Autodesk Inventor part; units mm, degrees
ref_plane "作業平面1" through (0, 0, 14) normal (0, 0, 1) x (-0.9659, -0.2588, 0)
ref_plane "YZ Plane" through (0, 0, 0) normal (1, 0, 0) x (0, 1, 0)
ref_plane "XZ Plane" through (0, 0, 0) normal (0, 1, 0) x (-1, 0, 0)
ref_plane "作業平面1" through (0, 0, 14) normal (0, 0, 1) x (-0.9659, -0.2588, 0)
sketch "スケッチ14" plane through (0, 0, 0) normal (0, 0, 1) x (1, 0, 0)
  circle A0 centre (0, 0) radius 25
  circle A1 centre (30, 0) radius 4.05
  line L0 (0, 25) -> (40, 25)
  line L1 (40, 25) -> (40, -25)
  line L2 (40, -25) -> (0, -25)
  line L3 (0, -25) -> (0, 25)
  line L4 (0, -25) -> (40, -10.4412)
  line L5 (0, 25) -> (40, 10.4412)
  line L6 (0.5157, 26.4168) -> (40.5157, 11.858)
  line L7 (0.5157, -26.4168) -> (40.5157, -11.858)
  circle A2 centre (0, 0) radius 6.5
  circle A3 centre (0, 0) radius 28
  line L8 (1.5417, 29.2358) -> (41.5417, 14.677)
  line L9 (1.5417, -29.2358) -> (41.5417, -14.677)
  point P0 (8.5505, -23.4923)
  point P1 (40, -12.0456)
  point P2 (40, 12.0456)
  point P3 (8.5505, 23.4923)
  point P4 (40, 15.2382)
  point P5 (9.5766, 26.3114)
  point P6 (9.5766, -26.3114)
  point P7 (40, -15.2382)
  dimension "d111" = 50
  dimension "d112" = 8.1
  dimension "d113" = 30
  dimension "d114" = 40
  dimension "d115" = 50
  dimension "d116" = 25
  dimension "d119" = 25
  dimension "d126" = 20
  dimension "d127" = 20
  dimension "d144" = 13
  dimension "d207" = 3
  dimension "d208" = 3
  dimension "d209" = 3
extrude "押し出し9" add sketch "スケッチ14" along normal blind 5 contours L3 A2 A0 | L0 L6 A0 | A0 L2 A3 L0 | L5 A0 L4 L3 A2 | A0 L5 | L4 A0 | A0 L7 L2 | L6 A3 L5 A0 | L6 L0 A3 | L5 A3 A1 L4 A0 | L7 A3 L2 | A0 L4 A3 L7 | A3 L0 L8 L1 L6 | L6 L1 L5 A3 | A3 L8 L0 | L5 L1 L4 A3 A1 | A3 L4 L1 L7 | L7 L1 L9 L2 A3 | L2 L9 A3
sketch "スケッチ15" plane through (0, 0, 0) normal (0, 0, -1) x (-1, 0, 0)
  circle A0 centre (-30, 0) radius 4.05
  circle A1 centre (-30, 0) radius 6.6
  point P0 (0, 0)
  dimension "d122" = 13.2
extrude "押し出し10" cut sketch "スケッチ15" against normal blind 2
sketch "スケッチ16" plane through (0, 0, 5) normal (0, 0, 1) x (1, 0, 0)
  circle A0 centre (30, 0) radius 4.05
  circle A1 centre (30, 0) radius 17
  arc A2 (8.5505, 23.4923) -> (8.5505, -23.4923) centre (0, 0) ccw
  circle A3 centre (0, 0) radius 25
  line L0 (40, -15.2382) -> (40, 15.2382)
  line L1 (40, 12.0456) -> (-0.2187, 26.6841)
  line L2 (40, -12.0456) -> (-2.6962, -27.5858)
  circle A4 centre (0, 0) radius 17.5
  line L3 (8.5505, 23.4923) -> (5.9854, 16.4446)
  line L4 (-17.5, 0) -> (-25, 0)
  line L5 (-2.7839, 19.6364) -> (32.5, 6.7941)
  line L6 (32.5, 6.7941) -> (32.5, -6.7941)
  line L7 (32.5, -6.7941) -> (-5.2613, -20.5381)
  line L8 (17.9474, 20.0721) -> (15.3823, 13.0244)
  point P0 (0, 25)
  point P1 (0, -25)
  dimension "d125" = 34
  dimension "d128" = 7.5
  dimension "d164" = 7.5
  dimension "d165" = 10
extrude "押し出し11" add sketch "スケッチ16" along normal blind 10 contours L8 L5 L3 A3 | A3 L1 L8 | L3 A4 L4 A2
sketch "スケッチ17" plane through (0, 0, 5) normal (0, 0, 1) x (1, 0, 0)
  circle A0 centre (30, 0) radius 4.05
  line L0 (0, 0) -> (30, 0)
  circle A1 centre (0, 0) radius 12.5
  line L1 (0, 0) -> (12.4415, 7.1831)
  point P0 (10.8253, 6.25)
  point P1 (0, 12.5)
  point P2 (-10.8253, 6.25)
  point P3 (-10.8253, -6.25)
  point P4 (0, -12.5)
  point P5 (10.8253, -6.25)
  dimension "d131" = 25
  dimension "d132" = 30
  dimension "d135" = 360
hole "穴5" at (10.8253, 6.25, 5) at (0, 12.5, 5) at (-10.8253, 6.25, 5) at (-10.8253, -6.25, 5) at (0, -12.5, 5) at (10.8253, -6.25, 5) direction (0, 0, -1) diameter 3.2 end through all
sketch "スケッチ18" plane through (0, 0, 5) normal (0, 0, 1) x (1, 0, 0)
  circle A0 centre (30, 0) radius 4.05
  line L0 (0, 0) -> (30, 0)
  circle A1 centre (0, 0) radius 10.2
  point P0 (10.2, 0)
  point P1 (-5.1, 8.8335)
  point P2 (-5.1, -8.8335)
  dimension "d145" = 20.4
  dimension "d148" = 360
hole "穴6" at (10.2, 0, 5) at (-5.1, 8.8335, 5) at (-5.1, -8.8335, 5) direction (0, 0, -1) diameter 4.2 end through all
sketch "スケッチ19" plane through (0, 0, 5) normal (0, 0, 1) x (1, 0, 0)
  circle A0 centre (0, 12.5) radius 1.6
  circle A1 centre (0, 0) radius 12.5
  circle A2 centre (0, 12.5) radius 3
  circle A3 centre (-10.8253, 6.25) radius 3
  circle A4 centre (-10.8253, -6.25) radius 3
  circle A5 centre (0, -12.5) radius 3
  circle A6 centre (10.8253, -6.25) radius 3
  circle A7 centre (10.8253, 6.25) radius 3
  dimension "d157" = 6
  dimension "d160" = 360
extrude "押し出し12" cut sketch "スケッチ19" against normal blind 3 contours A0 A1 | A0 A1 A2 | A1 A0 | A0 A1 A2 | A3 A1 | A1 A3 | A7 A1 | A1 A7 | A4 A1 | A1 A4 | A6 A1 | A1 A6 | A5 A1 | A1 A5
sketch "スケッチ20" plane through (0, 0, 15) normal (0, 0, 1) x (1, 0, 0)
  line L0 (17.9474, 20.0721) -> (8.5505, 23.4923)
  line L1 (17.9474, 20.0721) -> (15.3823, 13.0244)
  line L2 (15.3823, 13.0244) -> (5.9854, 16.4446)
  line L3 (5.9854, 16.4446) -> (8.5505, 23.4923)
  line L4 (0, 0) -> (0, 30.7788)
  circle A0 centre (0, 0) radius 21.25
  circle A1 centre (0, 0) radius 25
  point P0 (11.9664, 18.2584)
  point P1 (0, 21.25)
  point P2 (-10.625, 18.403)
  point P3 (-18.403, 10.625)
  point P4 (-21.25, 0)
  point P5 (-18.403, -10.625)
  point P6 (-10.625, -18.403)
  point P7 (0, -21.25)
  point P8 (10.625, -18.403)
  point P9 (18.403, -10.625)
  point P10 (21.25, 0)
  point P11 (18.403, 10.625)
  point P12 (10.625, 18.403)
  dimension "d167" = 7.5
  dimension "d168" = 5
  dimension "d169" = 3.75
  dimension "d170" = 3.75
  dimension "d171" = 50
  dimension "d174" = 360
hole "穴7" at (11.9664, 18.2584, 15) at (0, 21.25, 15) at (-10.625, 18.403, 15) at (-18.403, 10.625, 15) direction (0, 0, -1) diameter 2.459 end through all
sketch "スケッチ21" plane through (0, 0, 15) normal (0, 0, 1) x (1, 0, 0)
  circle A0 centre (0, 0) radius 25
  line L0 (40, -15.2382) -> (40, 15.2382)
  line L1 (40, 12.0456) -> (40, -12.0456)
  line L2 (8.5505, -23.4923) -> (40, -12.0456)
  line L3 (40, -12.0456) -> (8.5505, -23.4923)
  line L4 (40, 12.0456) -> (8.5505, 23.4923)
  line L5 (40, 0) -> (-25, 0)
  circle A1 centre (0, 0) radius 16
  circle A2 centre (30, 0) radius 4.05
  circle A3 centre (30, 0) radius 4.05
  line L6 (9.2345, 25.3717) -> (42, 13.4461)
  line L7 (42, 13.4461) -> (42, -13.4461)
  line L8 (42, -13.4461) -> (9.2345, -25.3717)
  circle A4 centre (0, 0) radius 27
  line L9 (40, 15.2382) -> (40, -15.2382)
  point P0 (40, 14.174)
  point P1 (9.2345, 25.3717)
  point P2 (9.2345, -25.3717)
  point P3 (40, -14.174)
  dimension "d183" = 32
  dimension "d184" = 8.1
  dimension "d210" = 2
  dimension "d211" = 2
extrude "押し出し13" add sketch "スケッチ21" along normal blind 5 contours L5 A1 A0 | L5 A2 A4 L2 A0 | A0 L5 A1 | A0 L4 A4 A2 L5 | A0 L2 A4 L4 | A4 L6 L0 L4 | L4 L0 L5 A2 A4 | A4 A2 L5 L0 L2 | L2 L0 L8 A4
sketch "スケッチ22" plane through (0, 0, 20) normal (0, 0, 1) x (1, 0, 0)
  circle A0 centre (0, 21.25) radius 1.2295
  circle A1 centre (0, 0) radius 21.25
  circle A2 centre (-10.625, 18.403) radius 1.2295
  circle A3 centre (-18.403, 10.625) radius 1.2295
  circle A4 centre (11.9664, 18.2584) radius 1.2295
  line L0 (-17.5, 0) -> (-25, 0)
  line L1 (-25, 0) -> (40, 0)
  line L2 (40, -15.2382) -> (40, 15.2382)
  point P0 (40, -12.0456)
  point P1 (40, 12.0456)
  point P2 (0, -21.25)
  point P3 (-10.625, -18.403)
  point P4 (-18.403, -10.625)
  point P5 (11.9664, -18.2584)
  point P6 (-21.25, 0)
  point P7 (-18.403, 10.625)
  point P8 (-21.25, 0)
  point P9 (-18.403, -10.625)
  point P10 (-10.625, -18.403)
  point P11 (0, -21.25)
  point P12 (10.625, -18.403)
  point P13 (18.403, -10.625)
  point P14 (21.25, 0)
  point P15 (18.403, 10.625)
  point P16 (10.625, 18.403)
  point P17 (0, 21.25)
  dimension "d215" = 360
hole "穴8" at (10.625, -18.403, 20) at (0, -21.25, 20) at (-10.625, -18.403, 20) at (-18.403, -10.625, 20) at (-18.403, 10.625, 20) at (-21.25, 0, 20) at (-10.625, 18.403, 20) at (0, 21.25, 20) at (10.625, 18.403, 20) direction (0, 0, -1) diameter 3.2 end through all
sketch "スケッチ23" plane through (0, 0, 0) normal (0, 0, -1) x (-1, 0, 0)
  line L0 (46.3543, -34.5724) -> (-56.544, -34.5724)
  line L1 (-56.544, -34.5724) -> (-56.544, 32.2069)
  line L2 (-56.544, 32.2069) -> (46.3543, 32.2069)
  line L3 (46.3543, 32.2069) -> (46.3543, -34.5724)
  point P0 (0, 0)
extrude "押し出し14" cut sketch "スケッチ23" against normal blind 15
sketch "スケッチ24" plane through (0, 0, 20) normal (0, 0, 1) x (1, 0, 0)
  circle A0 centre (0, 21.25) radius 1.6
  circle A1 centre (0, 21.25) radius 3
  circle A2 centre (-10.625, 18.403) radius 1.6
  circle A3 centre (-10.625, 18.403) radius 3
  circle A4 centre (-18.403, 10.625) radius 1.6
  circle A5 centre (-18.403, 10.625) radius 3
  line L0 (0, 0) -> (-8.2063, 0)
  circle A6 centre (0, -21.25) radius 3
  circle A7 centre (-10.625, -18.403) radius 3
  circle A8 centre (-18.403, -10.625) radius 3
  circle A9 centre (-21.25, -0.0076) radius 3
  circle A10 centre (0, 0) radius 21.25
  circle A11 centre (10.625, 18.403) radius 1.6
  circle A12 centre (10.625, 18.403) radius 3
  circle A13 centre (10.625, -18.403) radius 1.6
  circle A14 centre (10.625, -18.403) radius 3
  dimension "d198" = 6
  dimension "d199" = 6
  dimension "d200" = 6
  dimension "d203" = 6
  dimension "d217" = 6
  dimension "d218" = 6
extrude "押し出し15" cut sketch "スケッチ24" against normal blind 3 contours A0 A10 | A0 A10 A1 | A10 A0 | A0 A10 A1 | A10 A2 A3 | A3 A10 A2 | A12 A10 A11 | A10 A11 A12 | A10 A2 | A2 A10 | A10 A4 A5 | A5 A10 A4 | A14 A10 A13 | A10 A13 A14 | A10 A9 | A9 A10 | A10 A6 | A6 A10 | A10 A8 | A8 A10 | A10 A7 | A7 A10
fillet "フィレット10" radius 18 2 edges at (40, 14.174, 17.5) (40, -14.174, 17.5)
properties part number "RP_Thigh-Base-Cover" material "アルミニウム 6061"
Input: part model. Units: mm. Frame: model coordinates. A direction names the side the tool comes from. Give positions to 0.01 mm unless a question says otherwise; leave off trailing zeros. Write each loop counter-clockwise with the first axis right and the second up, starting at its lowest first coordinate (ties: lowest second). Pieces come first, ordered by that corner, then holes.
Q1. Section A-A, the plane x = 32.5. Output: boundary loops of the cut face in (y, z), plus the area to 3 significant figures.
Q2. Section D-D, the plane x = 19. Output: boundary loops of the cut face in (y, z).
Q3. Section C-C, the plane x = 5. Output: boundary loops of the cut face in (y, z).
Q4. Set-up query: faces 1 (the face through (-24.247, 0.124, 18.521)), 2 (the face through (-9.651, -17.133, 15.986)). Return all of +Z, -Z, +X, -X, +Y, -Y with unobstructed straight access to the full face (end or side cutting, diameter ignored); none if empty.
Q5. Pull-direction query (X, two-part tool) for faces 3 (the face through (13, -12, 15)), 4 (the face through (12, 17, 17)), 5 (the face through (18.83, -21.88, 17.46)); classes: pulls with the +X half, pulls with the -X half, needs draft (parallel to the pull), parting line crosses it, or undercut.
Q6. Section B-B, the plane z = 18.55. State how many separate pieces and enclosed holes the cut face has, plus the area to 3 significant figures.
Q7. Material intervals for probe 1 along Y at (x, z) = (0, 16); probe 2 along X at (y, z) = (1, 18.1); probe 3 along X at (y, z) = (-8.5, 17.9), sorted ascending.
Q8. First-contact query: P1, Ø5.5, axis at x = 10.625, y = 18.403, coming from the +Z side; P2, Ø1.5, axis at x = -2.5, z = 18, coming from the -Y side; P3, Ø2, axis at y = 15, z = 18.5, coming from the +X side. Flat tips, straight axial feed; report the tip coordinate or a pass-through.
Filled in:
1. outline: (-16.19, 15) - (-3.19, 15) - (-3.19, 20) - (-16.19, 20) - close; (3.19, 15) - (16.19, 15) - (16.19, 20) - (3.19, 20) - close
1. area: 130 mm2
2. outline: (-21.82, 15) - (21.82, 15) - (21.82, 20) - (-21.82, 20) - close
3. outline: (-26.53, 15) - (-15.2, 15) - (-15.2, 20) - (-26.53, 20) - close; (15.2, 15) - (26.53, 15) - (26.53, 20) - (15.2, 20) - close
4. face 1: +Z
4. face 2: +Z, -Z
5. face 3: needs draft
5. face 4: undercut
5. face 5: pulls with the +X half
6. separate pieces: 1
6. enclosed holes: 11
6. area: 1,680 mm2
7. probe 1: y = -27 to -22.85, -19.65 to -16, 16 to 19.65, 22.85 to 27
7. probe 2: x = -26.98 to -24.08, -18.42 to -15.97, 15.97 to 26.08, 33.92 to 40
7. probe 3: x = -25.63 to -20.52, -16.29 to -13.56, 13.56 to 38.61
8. P1: stops at z = 17
8. P2: stops at y = -26.94
8. P3: stops at x = 35.02
